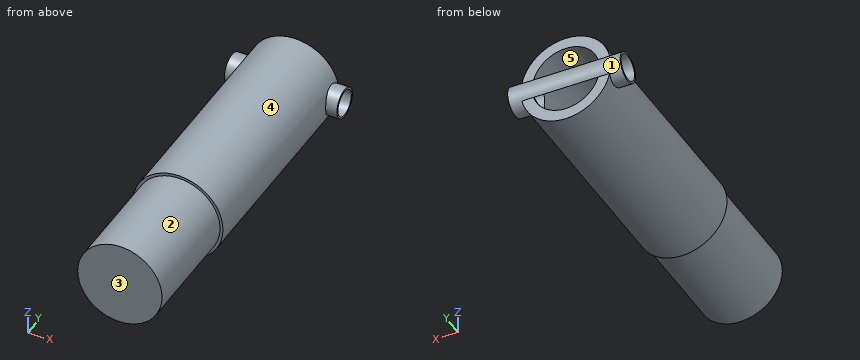
Autodesk Inventor part; units mm, degrees
ref_plane "YZ Plane" through (0, 0, 0) normal (1, 0, 0) x (0, 1, 0)
ref_plane "XZ Plane" through (0, 0, 0) normal (0, 1, 0) x (-1, 0, 0)
ref_plane "XY Plane" through (0, 0, 0) normal (0, 0, 1) x (1, 0, 0)
sketch "Sketch1" plane through (0, 0, 0) normal (0, 1, 0) x (-1, 0, 0)
  circle A0 centre (0, 0) radius 37.5
  dimension "d0" = 75
extrude "Extrusion1" add sketch "Sketch1" along normal blind 300
sketch "Sketch2" plane through (0, 0, 0) normal (1, 0, 0) x (0, 1, 0)
  circle A0 centre (290, 0) radius 13.25
  line L0 (0, -37.5) -> (0, 37.5)
  point P0 (0, 0)
  dimension "d3" = 290
  dimension "d4" = 26.5
extrude "Extrusion2" add sketch "Sketch2" along normal mid plane 100
sketch "Sketch4" plane through (0, 300, 0) normal (0, 1, 0) x (1, 0, 0)
  circle A0 centre (0, 0) radius 40
  dimension "d9" = 80
extrude "Extrusion4" add sketch "Sketch4" against normal blind 200
sketch "Sketch5" plane through (0, 300, 0) normal (0, 1, 0) x (1, 0, 0)
  circle A0 centre (0, 0) radius 30
  dimension "d12" = 60
extrude "Extrusion5" cut sketch "Sketch5" against normal blind 250
sketch "Sketch6" plane through (50, 290, 0) normal (1, 0, 0) x (0, 0, -1)
  circle A0 centre (0, 0) radius 13.25
  point P0 (0, -290)
hole "Hole1" at (50, 290, 0) direction (-1, 0, 0) diameter 23 end through all
properties part number "Water pump"
Model file for the job. Use its own axes, mm. Face numbers are marked on the shaded views. A direction names the side the tool comes from. Give positions to 0.01 mm unless a question says otherwise; leave off trailing zeros. Loops run counter-clockwise (first coordinate to the right, second up) from the corner with the lowest first, then second, coordinate; pieces in that order, holes last. Notation, with made-up numbers: (62.25, 28) -> (80.25, 28) arc R23 ccw to (80.25, 67) -> close; hole circle Ø4 at (37.5, -38). An arc over 180 degrees is marked (long way). Write each question's results on one line, items separated by ' | '.
(1) Cut at A-A on z = 0. List the corners of the cut face in (x, y).
Geometry results:
outline: (-50, 276.75) -> (-40, 276.75) -> (-40, 100) -> (-37.5, 100) -> (-37.5, 0) -> (37.5, 0) -> (37.5, 100) -> (40, 100) -> (40, 276.75) -> (50, 276.75) -> (50, 278.5) -> (30, 278.5) -> (30, 50) -> (-30, 50) -> (-30, 278.5) -> (-50, 278.5) -> close; (-50, 301.5) -> (50, 301.5) -> (50, 303.25) -> (-50, 303.25) -> close
(2) Pull direction Z, two halves, no side cores. Call the marked faces 3, 4 and 5: released by +Z, released by -Z, zero draft, split by the parting line, or undercut.
Geometry results:
face 3: zero draft | face 4: split by the parting line | face 5: undercut
(3) Cut at C-C on y = 290. List the corners of the cut face in (x, z), and give its area (3 significant figures).
Geometry results:
outline: (-50, -13.25) -> (-37.74, -13.25) arc R40 ccw to (37.74, -13.25) -> (50, -13.25) -> (50, -11.5) -> (27.71, -11.5) arc R30 cw to (-27.71, -11.5) -> (-50, -11.5) -> close; (-50, 11.5) -> (-27.71, 11.5) arc R30 cw to (27.71, 11.5) -> (50, 11.5) -> (50, 13.25) -> (37.74, 13.25) arc R40 ccw to (-37.74, 13.25) -> (-50, 13.25) -> close | area: 1,810 mm²
(4) Cut at D-D on z = -22.5. List the corners of the cut face in (x, y).
Geometry results:
outline: (-33.07, 100) -> (-30, 100) -> (-30, 0) -> (30, 0) -> (30, 100) -> (33.07, 100) -> (33.07, 300) -> (19.84, 300) -> (19.84, 50) -> (-19.84, 50) -> (-19.84, 300) -> (-33.07, 300) -> close
(5) Probe line 1 along X through (y, z) = (126, 0); line 2 along Y through (x, z) = (15.5, -6.5); line 3 along Y through (x, z) = (15, 0). List the from-to ranges inside material, lowest first.
Geometry results:
line 1: x = -40 to -30, 30 to 40 | line 2: y = 0 to 50, 300 to 301.55 | line 3: y = 0 to 50, 301.5 to 303.25
(6) Cut at B-B on x = 0. List the corners of the cut face in (y, z).
Geometry results:
outline: (0, -37.5) -> (100, -37.5) -> (100, -40) -> (300, -40) -> (300, -30) -> (50, -30) -> (50, 30) -> (300, 30) -> (300, 40) -> (100, 40) -> (100, 37.5) -> (0, 37.5) -> close; (300, -8.69) arc R13.25 ccw to (300, 8.69) -> (300, 5.68) arc R11.5 cw to (300, -5.68) -> close
(7) Tool access for the marked faces 1 and 2: list every direction of +Z, -Z, +X, -X, +Y, -Y with a clear straight run to the whole face (end or side of a thin tool).
Geometry results:
face 1: none | face 2: -Y
(8) Flat gauge pins, fed straight in: pin 1 Ø3 at (y, z) = (127, -29) entering from +X; pin 2 Ø8 at (x, z) = (-9.5, 10.5) entering from +Y; pin 3 Ø10 at (x, y) = (20, 205.5) entering from +Z. Where does each tip first touch, or does it go through?
Geometry results:
pin 1: stops at x = 29.05 | pin 2: stops at y = 301.55 | pin 3: stops at z = 37.08
